from build123d import *

# Parameters (mm, degrees)
BOSS_EXTRUDE1_DEPTH = 31.75
SKETCH19_W          = 15.860402013
SKETCH19_H          = 31.75
BOSS_EXTRUDE7_DEPTH = 2
SKETCH23_W          = 15.860402013
SKETCH23_H          = 2
BOSS_EXTRUDE8_DEPTH = 25
SKETCH24_R          = 1.27
CUT_EXTRUDE1_DEPTH  = 2.54


with BuildPart() as part:
    # Sketch2 → Boss-Extrude1 (new body)
    with BuildSketch(Plane.XY):
        with BuildLine():
            Line((-50.375618534, 45.609862895), (-50.351188886, 46.309436474))
            ThreePointArc((-50.351188886, 46.309436474), (-50.565618587, 46.88295476), (-51.12278195, 47.136868733))
            Line((-51.12278195, 47.136868733), (-55.780902554, 47.299533889))
            Line((-55.780902554, 47.299533889), (-47.850701548, 47.299533889))
            Line((-47.850701548, 47.299533889), (-47.850701548, 40.900752235))
            Line((-47.850701548, 40.900752235), (-48.952946324, 40.900752235))
            ThreePointArc((-48.952946324, 40.900752235), (-50.100996621, 41.129113637), (-51.074266668, 41.779431891))
            Line((-51.074266668, 41.779431891), (-53.375146928, 44.080312152))
            ThreePointArc((-53.375146928, 44.080312152), (-53.536830204, 44.931922499), (-52.803734096, 45.394471696))
            Line((-52.803734096, 45.394471696), (-50.685905631, 45.320515496))
            ThreePointArc((-50.685905631, 45.320515496), (-50.470836274, 45.400926634), (-50.375618534, 45.609862895))
        make_face()
    boss_extrude1 = extrude(amount=BOSS_EXTRUDE1_DEPTH)

    # Mirror2: Boss-Extrude1 across plane
    add(boss_extrude1.mirror(Plane(origin=(-47.850701548, 40.900752235, 31.75), x_dir=(0, 0, 1), z_dir=(-1, 0, 0))))

    # Sketch19 → Boss-Extrude7 (add)
    with BuildSketch(Plane(origin=(0, 47.299533889, 0), x_dir=(1, 0, 0), z_dir=(0, 1, 0))):
        with Locations((-47.850701548, -15.875)):
            Rectangle(SKETCH19_W, SKETCH19_H)
    extrude(amount=BOSS_EXTRUDE7_DEPTH)

    # Sketch23 → Boss-Extrude8 (add)
    with BuildSketch(Plane(origin=(0, 49.299533889, 0), x_dir=(1, 0, 0), z_dir=(0, 1, 0))):
        with Locations((-47.850701548, -28.75)):
            Rectangle(SKETCH23_W, SKETCH23_H)
    extrude(amount=BOSS_EXTRUDE8_DEPTH)

    # Sketch24 → Cut-Extrude1 (cut)
    with BuildSketch(Plane(origin=(0, 0, 27.75), x_dir=(-1, 0, 0), z_dir=(0, 0, -1))):
        with Locations((47.850701548, 67.949533889)):
            Circle(SKETCH24_R)
    extrude(amount=-CUT_EXTRUDE1_DEPTH, mode=Mode.SUBTRACT)


solid = part.part
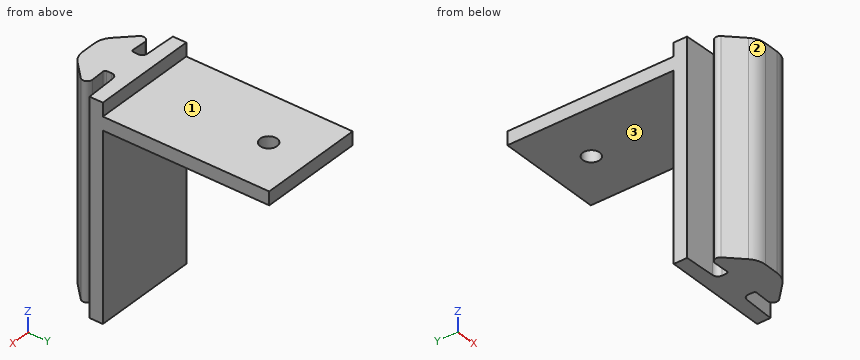
Verification items for the finished model (mm, model axes). Face numbers are marked on the shaded views. A direction names the side the tool comes from. Round coordinates to 2 decimals unless told otherwise and drop trailing zeros. Loops run counter-clockwise (first coordinate to the right, second up) from the corner with the lowest first, then second, coordinate; pieces in that order, holes last. Notation, with made-up numbers: (-30.75, 42) - (2.25, 42) arc R13 ccw to (2.25, 66) - close; hole circle Ø7 at (8, 52). An arc over 180 degrees is marked (long way). Answer in a Markdown table with one row per item. Add a question column.
Q1. Tool access check on the marked faces 1, 2 and 3. Record the directions out of +Z, -Z, +X, -X, +Y, -Y that give a thin tool (end or side, any length) a straight path to the whole face; none if there is none.
Q2. Material ranges on line 1 (Y direction, x = -47.5, z = 18); line 2 (Z direction, x = -54.5, y = 72.5); line 3 (Y direction, x = -43.25, z = 25), recorded low to high.
Q3. Gauge pin test, flat ends, axial feed: pin 1 (2 mm diameter, centred on x = -54, y = 64.5, fed in from +Z); pin 2 (5 mm diameter, centred on x = -47, z = 12.5, fed in from +Y); pin 3 (1.5 mm diameter, centred on x = -47.85, y = 67.95, fed in from +Z). Record the tip position at first contact, or that the pin passes through.
Q4. Section check D-D on z = 28.5. Enter the section's corners in (x, y).
Q5. Section check B-B on z = 19. Enter the section's corners in (x, y), plus the area to 3 significant figures.
Q6. Section check A-A on y = 68.5. Enter the section's corners in (x, z), plus the area to 3 significant figures.
Q7. Section check C-C on x = -41.25. Enter the section's corners in (y, z), plus the area to 3 significant figures.
Found:
| question | item | result |
|---|---|---|
| 1 | face 1 | +Z, +X, -X, +Y |
| 1 | face 2 | +Z, -Z, -X, -Y |
| 1 | face 3 | -Z, +X, -X, +Y |
| 2 | line 1 | y = 40.9 to 49.3 |
| 2 | line 2 | z = 27.75 to 29.75 |
| 2 | line 3 | y = 43.16 to 45.38, 47.18 to 49.3 |
| 3 | pin 1 | stops at z = 29.75 |
| 3 | pin 2 | stops at y = 49.3 |
| 3 | pin 3 | passes through |
| 4 | outline | (-55.78, 47.3) - (-51.12, 47.14) arc R0.8 cw to (-50.35, 46.31) - (-50.38, 45.61) arc R0.3 cw to (-50.69, 45.32) - (-52.8, 45.39) arc R0.77 ccw to (-53.38, 44.08) - (-51.07, 41.78) arc R3 ccw to (-48.95, 40.9) - (-46.75, 40.9) arc R3 ccw to (-44.63, 41.78) - (-42.33, 44.08) arc R0.77 ccw to (-42.9, 45.39) - (-45.02, 45.32) arc R0.3 cw to (-45.33, 45.61) - (-45.35, 46.31) arc R0.8 cw to (-44.58, 47.14) - (-39.92, 47.3) - (-39.92, 74.3) - (-55.78, 74.3) - close; hole circle Ø2.54 at (-47.85, 67.95) |
| 5 | outline | (-55.78, 47.3) - (-51.12, 47.14) arc R0.8 cw to (-50.35, 46.31) - (-50.38, 45.61) arc R0.3 cw to (-50.69, 45.32) - (-52.8, 45.39) arc R0.77 ccw to (-53.38, 44.08) - (-51.07, 41.78) arc R3 ccw to (-48.95, 40.9) - (-46.75, 40.9) arc R3 ccw to (-44.63, 41.78) - (-42.33, 44.08) arc R0.77 ccw to (-42.9, 45.39) - (-45.02, 45.32) arc R0.3 cw to (-45.33, 45.61) - (-45.35, 46.31) arc R0.8 cw to (-44.58, 47.14) - (-39.92, 47.3) - (-39.92, 49.3) - (-55.78, 49.3) - close |
| 5 | area | 81.8 mm² |
| 6 | outline | (-55.78, 27.75) - (-49, 27.75) - (-49, 29.75) - (-55.78, 29.75) - close; (-46.71, 27.75) - (-39.92, 27.75) - (-39.92, 29.75) - (-46.71, 29.75) - close |
| 6 | area | 27.1 mm² |
| 7 | outline | (47.25, 0) - (49.3, 0) - (49.3, 27.75) - (74.3, 27.75) - (74.3, 29.75) - (49.3, 29.75) - (49.3, 31.75) - (47.25, 31.75) - close |
| 7 | area | 115 mm² |
